CAD build for the part. Positions are in the model's coordinates, mm. Face numbers are marked on the shaded views. A direction names the side the tool comes from. Coordinates: 2 decimals unless noted, no trailing zeros. Order: outer loops, then holes, each group sorted by start corner. A loop starts at its lowest first (then second) coordinate and runs counter-clockwise, first axis right, second up. Notation, with made-up numbers: (64.25, 42) - (92.25, 42) arc R20 ccw to (92.25, 73) - close; hole circle Ø11 at (68.25, 55.25). An arc over 180 degrees is marked (long way). Write each question's results on one line, items separated by ' | '. Start each with the question number.
Q1. Band-saw the part on A-A, the plane z = 0. Write the cut outline in (x, y), then the cut area to 4 significant figures.
Q2. Wall check: probe 1 along X at (y, z) = (-1.5, -27); probe 2 along Y at (x, z) = (46, 1); probe 3 along Z at (x, y) = (41, 11). Give the ranges that are in metal, low to high.
Q3. Pin check, flat tips, straight feed: P1, Ø4, axis at y = -20.5, z = 13.5, coming from the +X side; P2, Ø12, axis at y = 18, z = -21, coming from the +X side; P3, Ø4, axis at y = 48.5, z = -27.5, coming from the +X side. Stop position of each tip, or through.
Q4. Band-saw the part on C-C, the plane x = 107. Write the cut outline in (y, z), then the cut area to 3 significant figures.
Q5. Which spindle directions (+Z, -Z, +X, -X, +Y, -Y) get a long thin tool onto all of the face, cutting with end or side? Do the marked faces 1 and 2. Say none if no direction does.
Q6. Band-saw the part on D-D, the plane x = 22.5. Write the cut outline in (y, z), then the cut area to 3 significant figures.
```python
from build123d import *

# Parameters (mm, degrees)
F2_SIZE2 = 10
F2_SIZE  = 10
F3_SIZE  = 5


with BuildPart() as f1:
    # F0 (on Top) → F1 (revolve)
    with BuildSketch(Plane.XY):
        Polygon((0, 65), (0, 0), (120, 0), (120, 25), (102, 25), (30, 25), (30, 65), align=None)
    revolve(axis=Axis((60, 0, 0), (-1, 0, 0)))

    # F2
    f2_edges = [f1.edges().sort_by_distance(p)[0] for p in [
        (0, -65, 0),
    ]]
    chamfer(f2_edges, length=F2_SIZE, length2=F2_SIZE2)

    # F3
    f3_edges = [f1.edges().sort_by_distance(p)[0] for p in [
        (120, -25, 0),
    ]]
    chamfer(f3_edges, length=F3_SIZE)


solid = f1.part
```
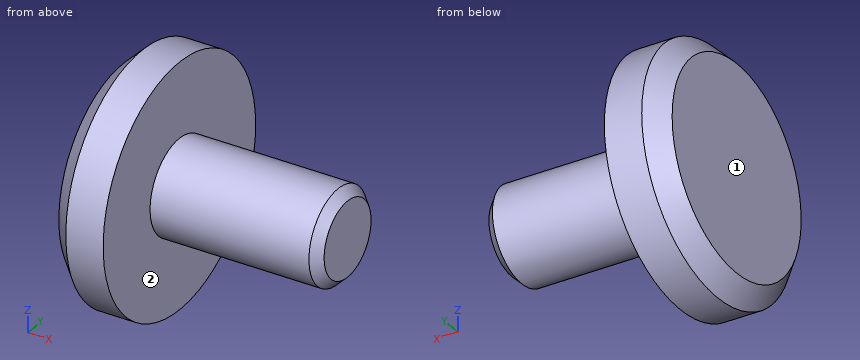
Results below:
1) outline: (0, -55) - (10, -65) - (30, -65) - (30, -25) - (115, -25) - (120, -20) - (120, 20) - (115, 25) - (30, 25) - (30, 65) - (10, 65) - (0, 55) - close | area: 8,275 mm²
2) probe 1: x = 0 to 30 | probe 2: y = -24.98 to 24.98 | probe 3: z = -22.45 to 22.45
3) P1: stops at x = 117.45 | P2: stops at x = 118.34 | P3: stops at x = 30
4) outline: circle Ø50 at (0, 0) | area: 1,960 mm²
5) face 1: +Z, -Z, -X, +Y, -Y | face 2: +X
6) outline: circle Ø130 at (0, 0) | area: 13,300 mm²
